Could you check a few things on this model? Use its own coordinates, in mm. Face numbers are marked on the shaded views. A direction names the side the tool comes from. Give positions to 0.01 mm unless a question says otherwise; leave off trailing zeros. Loops run counter-clockwise (first coordinate to the right, second up) from the corner with the lowest first, then second, coordinate; pieces in that order, holes last. Notation, with made-up numbers: (-20, 21.5) - (8, 21.5) arc R27 ccw to (8, 46.5) - close; hole circle Ø11 at (68.25, -8). An arc over 180 degrees is marked (long way). Write each question's results on one line, items separated by ' | '. Start each with the question number.
1) If I drill on probe 1 along Y at (x, z) = (17.75, 0); probe 2 along Y at (x, z) = (12, 3); probe 3 along Y at (x, z) = (11, 4.25), over which ranges is the centre line in solid material (lowest first)? Write a range as [from, to].
2) I want a section at B-B, the plane x = 15.25. Write out the boundary of the cut face in (y, z), and give its area (3 significant figures).
3) I want a section at C-C, the plane z = -1.5. Write out the boundary of the cut face in (x, y).
4) I want a section at A-A, the plane y = -20. Write out the boundary of the cut face in (x, z).
5) I'm going to push a flat-ended pin straight in: pin 1 (6.5 mm diameter, centred on y = 20, z = 0, fed in from +X). Where does the tip first touch, or does it pass through?
6) On a 3-axis mill with a long thin cutter (end or side, diameter ignored), from which of +Z, -Z, +X, -X, +Y, -Y can I reach the whole of each face in a straight line? I mean the marked faces 5 and 6. Say none if no direction works.
7) If we mould it in two halves opening along Y, with no side actions, what happens to the marked faces 1, 2, 3 and 4? For each: +Y half, -Y half, draft (parallel to the pull), parting line (faces both ways), or undercut.
8) I want a section at D-D, the plane y = 0.5. Write out the boundary of the cut face in (x, z), and give its area (3 significant figures).
from build123d import *

# Parameters (mm, degrees)
SKETCH1_W           = 20
SKETCH1_H           = 60
SKETCH1_R           = 4.1
SKETCH1_W_2         = 10
SKETCH1_H_2         = 20
BOSS_EXTRUDE1_DEPTH = 25


with BuildPart() as part:
    # Sketch1 → Boss-Extrude1 (new body)
    with BuildSketch(Plane(origin=(0, 0, 0), x_dir=(0, 0, -1), z_dir=(1, 0, 0))):
        Rectangle(SKETCH1_W, SKETCH1_H)
        with Locations((0, 20)):
            Circle(SKETCH1_R, mode=Mode.SUBTRACT)
        with Locations((0, -20)):
            Circle(SKETCH1_R, mode=Mode.SUBTRACT)
        Rectangle(SKETCH1_W_2, SKETCH1_H_2, mode=Mode.SUBTRACT)
    extrude(amount=BOSS_EXTRUDE1_DEPTH)


solid = part.part
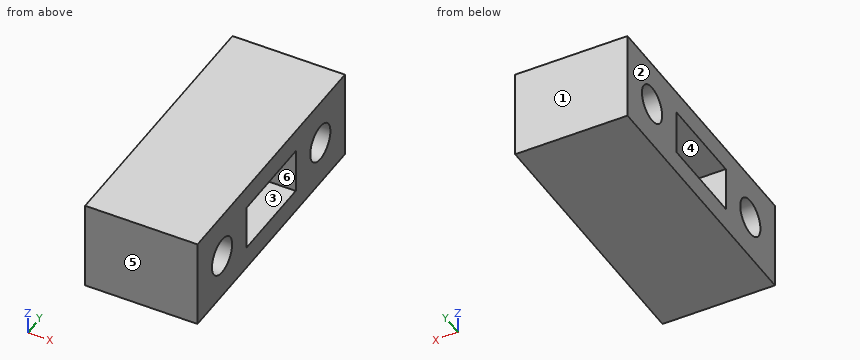
Answers:
1) probe 1: y = [-30, -24.1], [-15.9, -10], [10, 15.9], [24.1, 30] | probe 2: y = [-30, -22.79], [-17.21, -10], [10, 17.21], [22.79, 30] | probe 3: y = [-30, -10], [10, 30]
2) outline: (-30, -10) - (30, -10) - (30, 10) - (-30, 10) - close; hole circle Ø8.2 at (-20, 0); hole (-10, -5) - (10, -5) - (10, 5) - (-10, 5) - close; hole circle Ø8.2 at (20, 0) | area: 894 mm2
3) outline: (0, -30) - (25, -30) - (25, -23.82) - (0, -23.82) - close; (0, -16.18) - (25, -16.18) - (25, -10) - (0, -10) - close; (0, 10) - (25, 10) - (25, 16.18) - (0, 16.18) - close; (0, 23.82) - (25, 23.82) - (25, 30) - (0, 30) - close
4) outline: (0, -10) - (25, -10) - (25, -4.1) - (0, -4.1) - close; (0, 4.1) - (25, 4.1) - (25, 10) - (0, 10) - close
5) pin 1: passes through
6) face 5: +Z, -Z, +X, -X, -Y | face 6: +X, -X
7) face 1: +Y half | face 2: draft | face 3: undercut | face 4: undercut
8) outline: (0, -10) - (25, -10) - (25, -5) - (0, -5) - close; (0, 5) - (25, 5) - (25, 10) - (0, 10) - close | area: 250 mm2
